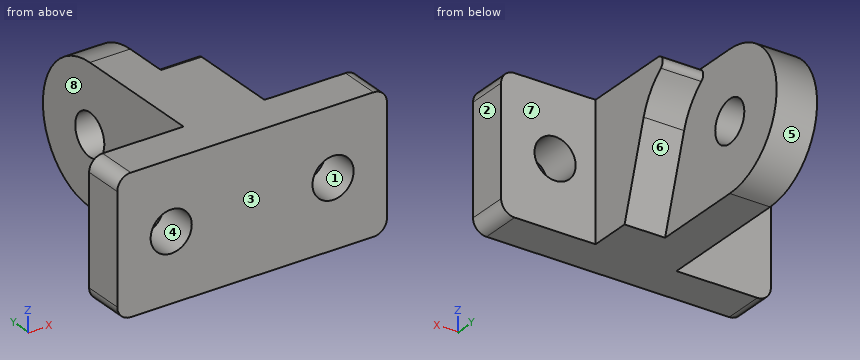
from build123d import *

# Parameters (mm, degrees)
SKETCH1_W           = 20
SKETCH1_H           = 10
SKETCH1_R           = 1.525
BOSS_EXTRUDE1_DEPTH = 3
SKETCH2_W           = 6
SKETCH2_H           = 10
BOSS_EXTRUDE2_DEPTH = 10
SKETCH3_R           = 5
SKETCH3_R_2         = 1.55
BOSS_EXTRUDE3_DEPTH = 3
CUT_EXTRUDE1_DEPTH  = 6
CUT_EXTRUDE2_START  = -3
SKETCH4_R           = 5
CUT_EXTRUDE2_DEPTH  = 3
FILLET2_R           = 1
CUT_EXTRUDE3_DEPTH  = 3
FILLET4_R           = 0.5
CUT_EXTRUDE4_DEPTH  = 3


with BuildPart() as part:
    # Sketch1 → Boss-Extrude1 (new body)
    with BuildSketch(Plane(origin=(0, 0, 0), x_dir=(1, 0, 0), z_dir=(0, 1, 0))):
        Rectangle(SKETCH1_W, SKETCH1_H)
        with Locations(Location((-6, 0, 0), (0, 0, 270))):
            Circle(SKETCH1_R, mode=Mode.SUBTRACT)
        with Locations(Location((6, 0, 0), (0, 0, 270))):
            Circle(SKETCH1_R, mode=Mode.SUBTRACT)
    extrude(amount=BOSS_EXTRUDE1_DEPTH)

    # Sketch2 → Boss-Extrude2 (add)
    with BuildSketch(Plane(origin=(0, 3, 0), x_dir=(1, 0, 0), z_dir=(0, 1, 0))):
        Rectangle(SKETCH2_W, SKETCH2_H)
    extrude(amount=BOSS_EXTRUDE2_DEPTH)

    # Sketch3 → Boss-Extrude3 (add)
    with BuildSketch(Plane.ZY.offset(3)):
        with Locations((0, 13)):
            Circle(SKETCH3_R)
        with Locations((0, 13)):
            Circle(SKETCH3_R_2, mode=Mode.SUBTRACT)
    extrude(amount=-BOSS_EXTRUDE3_DEPTH)

    # Sketch3_2 → Cut-Extrude1 (cut)
    with BuildSketch(Plane.ZY.offset(3)):
        with BuildLine():
            Line((-1.55, 13), (1.55, 13))
            ThreePointArc((1.55, 13), (0, 14.55), (-1.55, 13))
        make_face()
        with BuildLine():
            ThreePointArc((-1.55, 13), (0, 11.45), (1.55, 13))
            Line((1.55, 13), (-1.55, 13))
        make_face()
    extrude(amount=-CUT_EXTRUDE1_DEPTH, mode=Mode.SUBTRACT)

    # Sketch4 → Cut-Extrude2 (cut)
    with BuildSketch(Plane(origin=(3, 0, 0), x_dir=(0, 0, -1), z_dir=(1, 0, 0)).offset(CUT_EXTRUDE2_START)):
        with Locations((0, 13)):
            Circle(SKETCH4_R)
    extrude(amount=CUT_EXTRUDE2_DEPTH, mode=Mode.SUBTRACT)

    # Fillet2
    fillet2_edges = [part.edges().sort_by_distance(p)[0] for p in [
        (10, 1.5, 5),
        (-10, 1.5, 5),
        (-10, 1.5, -5),
        (10, 1.5, -5),
    ]]
    fillet(fillet2_edges, radius=FILLET2_R)

    # Sketch5 → Cut-Extrude3 (cut)
    with BuildSketch(Plane(origin=(3, 0, 0), x_dir=(0, 0, -1), z_dir=(1, 0, 0))):
        with BuildLine():
            Line((1.004987562, 8), (5, 8))
            Line((5, 8), (5, 14.099062692))
            Line((5, 14.099062692), (-5, 14.099062692))
            Line((-5, 14.099062692), (-5, 11.995012438))
            ThreePointArc((-5, 11.995012438), (-2.824900386, 8.753832574), (1.004987562, 8))
        make_face()
    extrude(amount=-CUT_EXTRUDE3_DEPTH, mode=Mode.SUBTRACT)

    # Fillet4
    fillet4_edges = [part.edges().sort_by_distance(p)[0] for p in [
        (1.5, 11.995012438, 5),
    ]]
    fillet(fillet4_edges, radius=FILLET4_R)

    # Sketch7 → Cut-Extrude4 (cut)
    with BuildSketch(Plane(origin=(3, 0, 0), x_dir=(0, 0, -1), z_dir=(1, 0, 0))):
        with BuildLine():
            Line((-1.517307451, 8.13093663), (5, 6.1))
            Line((5, 6.1), (5, 8))
            Line((5, 8), (1.004987562, 8))
            ThreePointArc((1.004987562, 8), (-0.264393679, 7.906857946), (-1.517307451, 8.13093663))
        make_face()
    extrude(amount=-CUT_EXTRUDE4_DEPTH, mode=Mode.SUBTRACT)


solid = part.part
Source: CAD feature listing. Evaluate the final solid. Frame: model axes, mm. Face numbers are marked on the shaded views. A direction names the side the tool comes from. Round coordinates to 2 decimals unless told otherwise and drop trailing zeros. Loops run counter-clockwise (first coordinate to the right, second up) from the corner with the lowest first, then second, coordinate; pieces in that order, holes last. Notation, with made-up numbers: M 71,69 L 102,69 A11 cw 102,79 Z; hole C 28,-23.5 d1. An arc over 180 degrees is marked long. Return JSON: item names as keys, results as strings. Group by question number.
1. Mould query, pull axis X, two halves, no side actions, for the marked faces 1, 2, 3 and 4. Classes: released by +X, released by -X, zero draft, split by the parting line, or undercut.
2. Section query A-A on y = 2.75. Output: boundary loops of the cut face in (x, z) (3 decimals), and give its area (3 significant figures).
3. Section query D-D on y = 13.25. Output: boundary loops of the cut face in (x, z).
4. Section query B-B on x = -6. Output: boundary loops of the cut face in (y, z) (3 decimals), and give its area (4 significant figures).
5. Reachability of the marked faces 5, 6, 7 and 8 from +Z, -Z, +X, -X, +Y, -Y: full face, straight path, thin tool, end or side. Return the list, or none.
6. Pin query (flat end, axial travel): pin 1 (1.5 mm diameter, centred on x = 0, y = 16, fed in from +Z); pin 2 (5 mm diameter, centred on y = 13, z = 2, fed in from -X); pin 3 (3.5 mm diameter, centred on x = -7.5, z = -0.5, fed in from +Y). Return the tip coordinate at first contact, or that it passes through.
7. Material intervals for line 1 along X through (y, z) = (0.9, 0) (3 decimals); line 2 along X through (y, z) = (4.5, -3.75); line 3 along Y through (x, z) = (6.75, 4), sorted ascending. Write a range as from..to.
8. Section query C-C on z = 0. Output: boundary loops of the cut face in (x, y) (3 decimals).
Checks:
{
 "1": {"face 1": "undercut", "face 2": "released by +X", "face 3": "zero draft", "face 4": "undercut"},
 "2": {"outline": "M -10,-4 A1 ccw -9,-5 L 9,-5 A1 ccw 10,-4 L 10,4 A1 ccw 9,5 L -9,5 A1 ccw -10,4 Z; hole C -6,0 d3.05; hole C 6,0 d3.05", "area": "185 mm²"},
 "3": {"outline": "M -3,-4.99 L 0,-4.99 L 0,-1.53 L -3,-1.53 Z; M -3,1.53 L 0,1.53 L 0,4.99 L -3,4.99 Z"},
 "4": {"outline": "M 0,-5 L 3,-5 L 3,-1.525 L 0,-1.525 Z; M 0,1.525 L 3,1.525 L 3,5 L 0,5 Z", "area": "20.85 mm²"},
 "5": {"face 5": "+X, -X, +Y", "face 6": "-Z, +X, +Y", "face 7": "+Z, -Z, +X, +Y", "face 8": "+Z, -Z, -X, +Y"},
 "6": {"pin 1": "stops at z = 4.47", "pin 2": "stops at x = -3", "pin 3": "stops at y = 3"},
 "7": {"line 1": "x = -10..-7.525, -4.475..4.475, 7.525..10", "line 2": "x = -3..3", "line 3": "y = 0..3"},
 "8": {"outline": "M -10,0 L -7.525,0 L -7.525,3 L -10,3 Z; M -4.475,0 L 4.475,0 L 4.475,3 L 3,3 L 3,7.658 L 0,7.658 L 0,11.45 L -3,11.45 L -3,3 L -4.475,3 Z; M -3,14.55 L 0,14.55 L 0,18 L -3,18 Z; M 7.525,0 L 10,0 L 10,3 L 7.525,3 Z"}
}
